```python
from build123d import *

# Parameters (mm, degrees)
SKETCH_1_W                  = 82
SKETCH_1_H                  = 63.5
EXTRUDE_1_DEPTH             = 16
CUT_EXTRUDE_1_DEPTH         = 83
SKETCH_15_W                 = 23.6
SKETCH_15_H                 = 14.711451884
CUT_EXTRUDE_4_DEPTH         = 7
SKETCH_16_W                 = 23.6
SKETCH_16_H                 = 10.67
CUT_EXTRUDE_5_DEPTH         = 9
SKETCH_17_R                 = 2.5
CUT_EXTRUDE_6_DEPTH         = 8
M4X0_72_D                   = 3.3
M4X0_72_DEPTH               = 10
M4X0_72_TIP                 = 0.991420021
CUT_EXTRUDE_7_DEPTH         = 4
SKETCH_26_R                 = 3.25
CUT_EXTRUDE_8_DEPTH         = 38
HOLE_WIZARD_M41_D           = 4.5
HOLE_WIZARD_M41_CBORE_D     = 8
HOLE_WIZARD_M41_CBORE_DEPTH = 4
CHAMFER_2_SIZE              = 1
CHAMFER_2_SIZE2             = 2
CHAMFER_2_PART_2_SIZE       = 1
CHAMFER_2_PART_2_SIZE2      = 2
CHAMFER_2_PART_3_SIZE       = 1
CHAMFER_2_PART_3_SIZE2      = 2
CUT_EXTRUDE_12_DEPTH        = 10.6
FILLET_1_R                  = 2


with BuildPart() as part:
    # Эскиз1 → Бобышка-Вытянуть1 (new body)
    with BuildSketch(Plane.XY):
        with Locations((41, -31.75)):
            Rectangle(SKETCH_1_W, SKETCH_1_H)
    extrude(amount=EXTRUDE_1_DEPTH)

    # Эскиз2 → Вырез-Вытянуть1 (cut, through all)
    with BuildSketch(Plane.ZY):
        Polygon((9, -10.67), (16, -14.711451884), (16, -48.788548116), (9, -52.83), align=None)
    extrude(amount=-CUT_EXTRUDE_1_DEPTH, mode=Mode.SUBTRACT)

    # Эскиз15 → Вырез-Вытянуть4 (cut)
    with BuildSketch(Plane.XY.offset(16)):
        with Locations((41, -56.144274058)):
            Rectangle(SKETCH_15_W, SKETCH_15_H)
    extrude(amount=-CUT_EXTRUDE_4_DEPTH, mode=Mode.SUBTRACT)

    # Эскиз16 → Вырез-Вытянуть5 (cut)
    with BuildSketch(Plane.XY.offset(9)):
        with Locations((41, -58.165)):
            Rectangle(SKETCH_16_W, SKETCH_16_H)
    extrude(amount=-CUT_EXTRUDE_5_DEPTH, mode=Mode.SUBTRACT)

    # Эскиз17 → Вырез-Вытянуть6 (cut)
    with BuildSketch(Plane.XZ.offset(52.83)):
        with Locations((33.5, 5)):
            Circle(SKETCH_17_R)
        with Locations((48.5, 5)):
            Circle(SKETCH_17_R)
    extrude(amount=-CUT_EXTRUDE_6_DEPTH, mode=Mode.SUBTRACT)

    # Отверстие обработанное метчиком M4x0.72
    with Locations(Plane(origin=(0, -52.83, 0), x_dir=(-1, 0, 0), z_dir=(0, -1, 0))):
        with Locations((-41, -5)):
            Hole(M4X0_72_D / 2, depth=M4X0_72_DEPTH)
            with Locations((0, 0, -(M4X0_72_DEPTH + M4X0_72_TIP / 2))):  # 118° drill point
                Cone(0, M4X0_72_D / 2, M4X0_72_TIP, mode=Mode.SUBTRACT)

    # Эскиз25 → Вырез-Вытянуть7 (cut)
    with BuildSketch(Plane.XY.offset(9)):
        with BuildLine():
            Line((44.1, -18.711451884), (44.1, -25.711451884))
            ThreePointArc((44.1, -25.711451884), (41, -28.811451884), (37.9, -25.711451884))
            Line((37.9, -25.711451884), (37.9, -18.711451884))
            ThreePointArc((37.9, -18.711451884), (41, -15.611451884), (44.1, -18.711451884))
        make_face()
    extrude(amount=-CUT_EXTRUDE_7_DEPTH, mode=Mode.SUBTRACT)

    # Эскиз26 → Вырез-Вытянуть8 (cut)
    with BuildSketch(Plane(origin=(0, 0, 0), x_dir=(1, 0, 0), z_dir=(0, 1, 0))):
        with Locations((41, -4.5)):
            Circle(SKETCH_26_R)
    extrude(amount=-CUT_EXTRUDE_8_DEPTH, mode=Mode.SUBTRACT)

    # Цековка для винта с внутренним шестигранником M41 (through all)
    with Locations(Plane(origin=(30.759227947, 26.793365177, 16), x_dir=(-1, 0, 0), z_dir=(0, 0, 1))):
        with Locations((-46.240772053, 31.793365177), (-46.240772053, 85.293365177), (25.759227947, 85.293365177), (25.759227947, 31.793365177)):
            CounterBoreHole(HOLE_WIZARD_M41_D / 2, HOLE_WIZARD_M41_CBORE_D / 2, HOLE_WIZARD_M41_CBORE_DEPTH)

    # Фаска2
    chamfer_2_edges = [part.edges().sort_by_distance(p)[0] for p in [
        (41, -14.711451884, 16),
    ]]
    chamfer_2_side = [part.faces().sort_by_distance(p)[0] for p in [
        (41, -7.569889145, 16),
    ]]
    chamfer(chamfer_2_edges, length=CHAMFER_2_SIZE, length2=CHAMFER_2_SIZE2, reference=chamfer_2_side[0])

    # Фаска2 part 2
    chamfer_2_part_2_edges = [part.edges().sort_by_distance(p)[0] for p in [
        (67.4, -48.788548116, 16),
    ]]
    chamfer_2_part_2_side = [part.faces().sort_by_distance(p)[0] for p in [
        (66.127821531, -55.832096576, 16),
    ]]
    chamfer(chamfer_2_part_2_edges, length=CHAMFER_2_PART_2_SIZE, length2=CHAMFER_2_PART_2_SIZE2, reference=chamfer_2_part_2_side[0])

    # Фаска2 part 3
    chamfer_2_part_3_edges = [part.edges().sort_by_distance(p)[0] for p in [
        (14.6, -48.788548116, 16),
    ]]
    chamfer_2_part_3_side = [part.faces().sort_by_distance(p)[0] for p in [
        (15.872178469, -55.832096576, 16),
    ]]
    chamfer(chamfer_2_part_3_edges, length=CHAMFER_2_PART_3_SIZE, length2=CHAMFER_2_PART_3_SIZE2, reference=chamfer_2_part_3_side[0])

    # Эскиз32 → Вырез-Вытянуть12 (cut)
    with BuildSketch(Plane.XZ.offset(63.5)):
        with BuildLine():
            Line((29.5, 12.3), (25.5, 12.3))
            ThreePointArc((25.5, 12.3), (21.2, 8), (25.5, 3.7))
            Line((25.5, 3.7), (29.5, 3.7))
            Line((29.5, 3.7), (29.5, 12.3))
        make_face()
        with BuildLine():
            Line((52.5, 3.7), (56.5, 3.7))
            ThreePointArc((56.5, 3.7), (60.8, 8), (56.5, 12.3))
            Line((56.5, 12.3), (52.5, 12.3))
            Line((52.5, 12.3), (52.5, 3.7))
        make_face()
    extrude(amount=-CUT_EXTRUDE_12_DEPTH, mode=Mode.SUBTRACT)

    # Скругление1
    fillet_1_edges = [part.edges().sort_by_distance(p)[0] for p in [
        (29.2, -58.2, 12.3),
        (29.2, -58.2, 3.7),
        (52.8, -58.2, 3.7),
        (52.8, -58.2, 12.3),
    ]]
    fillet(fillet_1_edges, radius=FILLET_1_R)


solid = part.part
```
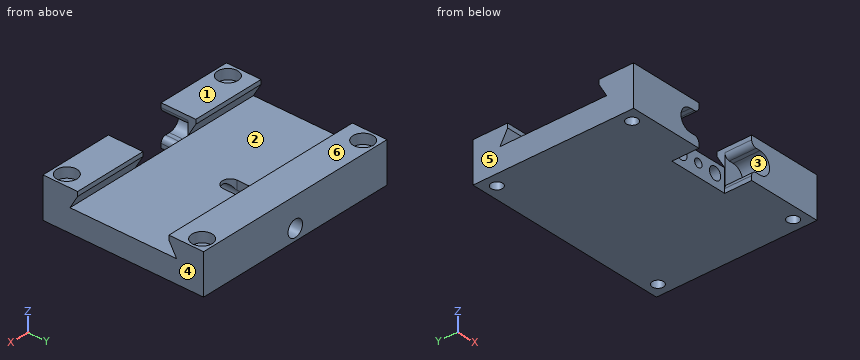
CAD build for the part. Positions are in the model's coordinates, mm. Face numbers are marked on the shaded views. A direction names the side the tool comes from. Coordinates: 2 decimals unless noted, no trailing zeros. Write each loop counter-clockwise with the first axis right and the second up, starting at its lowest first coordinate (ties: lowest second). Pieces come first, ordered by that corner, then holes.
(1) Cut at C-C, the plane z = 10.5. List the corners of the cut face in (x, y), and give its area (3 significant figures).
(2) Flat gauge pins, fed straight in: pin 1 (4 mm diameter, centred on x = 33, z = 6, fed in from -Y); pin 2 (2.5 mm diameter, centred on x = 55, z = 6.5, fed in from -Y); pin 3 (6 mm diameter, centred on x = 77, y = -58.5, fed in from -Z); pin 4 (4 mm diameter, centred on x = 58, y = -38, fed in from +Z). Where does each tip first touch, or does it go through?
(3) Cut at D-D, the plane x = 48.5. List the corners of the cut face in (y, z), and give its area (3 significant figures).
(4) 3-axis set-ups, long thin cutter, end or side, ignore diameter. For the marked faces 1 and 2: which of +Z, -Z, +X, -X, +Y, -Y reach the whole face in a straight line?
(5) Drill centre lines: probe 1 along Y at (x, z) = (5, 2); probe 2 along X at (y, z) = (-58.5, 14.5); probe 3 along X at (y, z) = (-52.5, 14.5). Where is each one in solid material? Low to high.
(6) Two-plate mould, pull along X, no slides. Class the marked faces 3, 4, 5 and 6: +X half, -X half, draft (parallel to the pull), parting line (faces both ways), or undercut.
(7) Cut at A-A, the plane y = -5. List the corners of the cut face in (x, z).
(8) Cut at B-B, the plane x = 77. List the corners of the cut face in (y, z).
Geometry says:
1. outline: (0, -63.5) - (22, -63.5) - (22, -52.9) - (29.2, -52.9) - (29.2, -51.96) - (0, -51.96) - close; (0, -11.54) - (82, -11.54) - (82, 0) - (0, 0) - close; (52.8, -52.9) - (60, -52.9) - (60, -63.5) - (82, -63.5) - (82, -51.96) - (52.8, -51.96) - close; hole circle Ø4.5 at (5, -58.5); hole circle Ø4.5 at (5, -5); hole circle Ø4.5 at (77, -58.5); hole circle Ø4.5 at (77, -5)
1. area: 1,400 mm2
2. pin 1: stops at y = -52.83
2. pin 2: stops at y = -52.9
2. pin 3: stops at z = 0
2. pin 4: stops at z = 9
3. outline: (-52.83, 0) - (0, 0) - (0, 16) - (-13.71, 16) - (-13.71, 14.27) - (-10.67, 9) - (-52.83, 9) - (-52.83, 7.5) - (-44.83, 7.5) - (-44.83, 2.5) - (-52.83, 2.5) - close
3. area: 523 mm2
4. face 1: +Z, +X, -X, +Y, -Y
4. face 2: +X, -X
5. probe 1: y = -63.5 to -60.75, -56.25 to -7.25, -2.75 to 0
5. probe 2: x = 0 to 1, 9 to 29.2, 52.8 to 73, 81 to 82
5. probe 3: x = 0 to 29.2, 52.8 to 82
6. face 3: undercut
6. face 4: +X half
6. face 5: -X half
6. face 6: draft
7. outline: (0, 0) - (2.75, 0) - (2.75, 12) - (1, 12) - (1, 16) - (0, 16) - close; (7.25, 0) - (74.75, 0) - (74.75, 12) - (73, 12) - (73, 16) - (9, 16) - (9, 12) - (7.25, 12) - close; (79.25, 0) - (82, 0) - (82, 16) - (81, 16) - (81, 12) - (79.25, 12) - close; hole circle Ø6.5 at (41, 4.5)
8. outline: (-63.5, 0) - (-60.75, 0) - (-60.75, 12) - (-62.5, 12) - (-62.5, 16) - (-63.5, 16) - close; (-56.25, 0) - (-7.25, 0) - (-7.25, 12) - (-9, 12) - (-9, 16) - (-13.71, 16) - (-13.71, 14.27) - (-10.67, 9) - (-52.83, 9) - (-49.79, 14.27) - (-49.79, 16) - (-54.5, 16) - (-54.5, 12) - (-56.25, 12) - close; (-2.75, 0) - (0, 0) - (0, 16) - (-1, 16) - (-1, 12) - (-2.75, 12) - close
